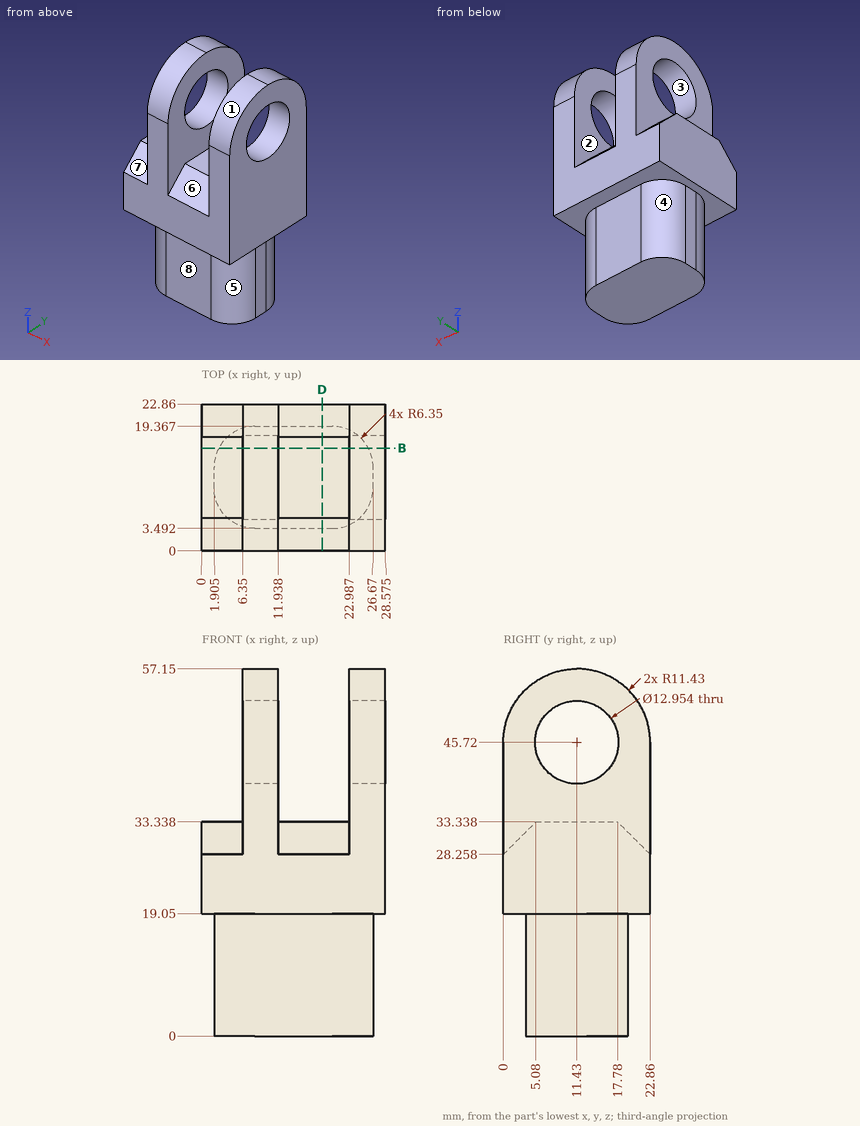
Geometry check sheet. Reference: drawing and pictorial views, mm from the part's lowest x, y, z. A direction names the side the tool comes from. Give positions to 0.01 mm unless a question says otherwise; leave off trailing zeros. Order: outer loops, then holes, each group sorted by start corner. A loop starts at its lowest first (then second) coordinate and runs counter-clockwise, first axis right, second up. Notation, with made-up numbers: M 40.5,17 L 56.5,17 A28 cw 56.5,53 Z; hole C 42.5,28 d4. An arc over 180 degrees is marked long. Answer in a Markdown table with one row per item.
1) Cross-section at B-B, the plane y = 16. Count the separate pieces of the cut face and the enclosed holes in it, plus the area to 3 significant figures.
Filled sheet:
| item | result |
|---|---|
| separate pieces | 3 |
| enclosed holes | 0 |
| area | 1,000 mm2 |
2) Access from +Z, -Z, +X, -X, +Y, -Y to the whole of each face (thin tool, end or side, straight path). Record for the marked faces 4, 5, 6, 7 and 8.
Filled sheet:
| item | result |
|---|---|
| face 4 | -Z, -X, +Y |
| face 5 | -Z, +X, -Y |
| face 6 | +Z, -Y |
| face 7 | +Z, -X, -Y |
| face 8 | -Z, +X, -X, -Y |
3) Release check for a two-part mould opening along Y. For the marked faces 1, 2 and 3 record: +Y half, -Y half, draft (parallel to the pull), parting line (faces both ways), or undercut.
Filled sheet:
| item | result |
|---|---|
| face 1 | -Y half |
| face 2 | draft |
| face 3 | undercut |
4) Cross-section at D-D, the plane x = 18.75. Enter the section's corners in (y, z).
Filled sheet:
| item | result |
|---|---|
| outline | M 0,19.05 L 3.49,19.05 L 3.49,0 L 19.37,0 L 19.37,19.05 L 22.86,19.05 L 22.86,28.26 L 17.78,33.34 L 5.08,33.34 L 0,28.26 Z |
5) Thickness scan on L1, parallel to Z at x = 10.55, y = 11.43; L2, parallel to X at y = 11.25, z = 7 (1 decimal); L3, parallel to Z at x = 17, y = 11.5. Record the ranges inside material, lowest first. Write a range as [from, to].
Filled sheet:
| item | result |
|---|---|
| L1 | z = [0, 39.24], [52.2, 57.15] |
| L2 | x = [1.9, 26.7] |
| L3 | z = [0, 33.34] |
6) Gauge pin test, flat ends, axial feed: P1, Ø3.5, axis at y = 11, z = 12, coming from the +X side; P2, Ø3.5, axis at x = 15, y = 13.5, coming from the +Z side; P3, Ø2, axis at x = 10.5, z = 14.5, coming from the +Y side; P4, Ø1.5, axis at x = 14.5, z = 45.5, coming from the +Y side. Record the tip position at first contact, or that the pin passes through.
Filled sheet:
| item | result |
|---|---|
| P1 | stops at x = 26.67 |
| P2 | stops at z = 33.34 |
| P3 | stops at y = 19.37 |
| P4 | passes through |
